Check sheet for the modelled part. Datum: model origin and axes. Units: mm. A direction names the side the tool comes from. Coordinates: 2 decimals unless noted, no trailing zeros. Write each loop counter-clockwise with the first axis right and the second up, starting at its lowest first coordinate (ties: lowest second). Pieces come first, ordered by that corner, then holes. Notation, with made-up numbers: M 36.25,-32 L 55.25,-32 A18 cw 55.25,-27 Z; hole C 86,50.25 d3. An arc over 180 degrees is marked long. Answer as CSV lines item,"result". Start each with the question number.
Q1. Sectioned sample at C-C, the plane y = 22. Record the cut outline in (x, z).
Q2. Sectioned sample at D-D, the plane x = 48. Record the cut outline in (y, z), then the cut area to 3 significant figures.
Q3. Sectioned sample at B-B, the plane x = -40. Record the cut outline in (y, z), then the cut area to 3 significant figures.
Q4. Depth check by flat-ended pin: pin 1 Ø8 at (x, z) = (135, 5) entering from -Y; pin 2 Ø10.5 at (x, y) = (0, 0) entering from -Z; pin 3 Ø9 at (x, y) = (-40, 0) entering from -Z; pin 4 Ø3 at (x, y) = (150, 0) entering from -Z. Enter the tip coordinate at first touch or a pass-through.
Q5. Access from +Z, -Z, +X, -X, +Y, -Y to the whole of each face (thin tool, end or side, straight path). Record for faces 4 (the flat face through (3, -3, 15)), 5 (the flat face through (91.08, 4.48, 9.86)), 6 (the flat face through (-24, 0, 8)).
Q6. Thickness scan on line 1 along Y through (x, z) = (0, 12.5); line 2 along Y through (x, z) = (0, 1.8); line 3 along Y through (x, z) = (52, 10.25). Record the ranges inside material, lowest first. Write a range as from..to.
Q7. Sectioned sample at A-A, the plane x = 0. Record the cut outline in (y, z).
Q8. Mould release check, pull along X, two halves, no side actions. Record for faces 1 (the flat face through (40, 10, 20)), 2 (the flat face through (150.1, -2.2, 4)), 3 (the cylindrical face through (-3.908, 29.614, 9.86)): pulls with the +X half, pulls with the -X half, needs draft (parallel to the pull), parting line crosses it, or undercut.
from build123d import *

# Parameters (mm, degrees)
SKETCH1_R           = 3.5
SKETCH1_R_2         = 2
BOSS_EXTRUDE1_DEPTH = 20
FILLET1_R           = 10
SKETCH2_R           = 2
CUT_EXTRUDE4_DEPTH  = 10
FILLET3_R           = 8.5
SKETCH3_R           = 6.5
CUT_EXTRUDE5_DEPTH  = 5
CUT_EXTRUDE7_START  = -5
SKETCH5_R           = 6.5
CUT_EXTRUDE7_DEPTH  = 5
SKETCH7_R           = 5
CUT_EXTRUDE8_DEPTH  = 4
CUT_EXTRUDE9_START  = -4
SKETCH8_R           = 5
CUT_EXTRUDE9_DEPTH  = 4


with BuildPart() as part:
    # Sketch1 → Boss-Extrude1 (new body)
    with BuildSketch(Plane.XY):
        with BuildLine():
            Line((-10.504774602, 27.019098406), (-43.939290476, 6.382161902))
            ThreePointArc((-43.939290476, 6.382161902), (-43.654129269, -6.54960604), (-32.5, 0))
            Line((-32.5, 0), (-17.320508076, 0))
            ThreePointArc((-17.320508076, 0), (0, -10), (17.320508076, 0))
            Line((17.320508076, 0), (142.5, 0))
            ThreePointArc((142.5, 0), (154.891549026, -5.685309853), (151.1193995, 7.4159925))
            Line((151.1193995, 7.4159925), (2.985065333, 29.77598))
            ThreePointArc((2.985065333, 29.77598), (-4.004573123, 29.594983902), (-10.504774602, 27.019098406))
        make_face()
        with BuildLine():
            ThreePointArc((12.1875, 10.748364701), (0, 16.25), (-12.1875, 10.748364701))
            ThreePointArc((-12.1875, 10.748364701), (-17.480391854, 10.416256555), (-17.8125, 15.709148409))
            ThreePointArc((-17.8125, 15.709148409), (0, 23.75), (17.8125, 15.709148409))
            ThreePointArc((17.8125, 15.709148409), (17.480391854, 10.416256555), (12.1875, 10.748364701))
        make_face(mode=Mode.SUBTRACT)
        with BuildLine():
            Line((44.021582733, 15.551547034), (64.021582733, 14.042107131))
            ThreePointArc((64.021582733, 14.042107131), (67.478730737, 10.020524397), (63.457148004, 6.563376394))
            Line((63.457148004, 6.563376394), (43.457148004, 8.072816297))
            ThreePointArc((43.457148004, 8.072816297), (40, 12.09439903), (44.021582733, 15.551547034))
        make_face(mode=Mode.SUBTRACT)
        with BuildLine():
            ThreePointArc((80.93587874, 5.244221712), (77.478730737, 9.265804446), (81.50031347, 12.722952449))
            Line((81.50031347, 12.722952449), (101.50031347, 11.213512546))
            ThreePointArc((101.50031347, 11.213512546), (104.957461474, 7.191929813), (100.93587874, 3.734781809))
            Line((100.93587874, 3.734781809), (80.93587874, 5.244221712))
        make_face(mode=Mode.SUBTRACT)
        Circle(SKETCH1_R, mode=Mode.SUBTRACT)
        with Locations((-40, 0)):
            Circle(SKETCH1_R_2, mode=Mode.SUBTRACT)
        with Locations((150, 0)):
            Circle(SKETCH1_R_2, mode=Mode.SUBTRACT)
    extrude(amount=BOSS_EXTRUDE1_DEPTH)

    # Fillet1
    fillet1_edges = [part.edges().sort_by_distance(p)[0] for p in [
        (-32.5, 0, 10),
        (142.5, 0, 10),
        (17.320508076, 0, 10),
        (-17.320508076, 0, 10),
    ]]
    fillet(fillet1_edges, radius=FILLET1_R)

    # Sketch2 → Cut-Extrude4 (cut)
    # profile 1 of 3: a face of its own
    with BuildSketch(Plane.XY.offset(20)):
        with BuildLine():
            ThreePointArc((-30, 0), (-30.37066789, 2.697399324), (-31.455192622, 5.194830784))
            ThreePointArc((-31.455192622, 5.194830784), (-34.377165478, 8.269445685), (-38.310752735, 9.856289549))
            Line((-38.310752735, 9.856289549), (-43.939290476, 6.382161902))
            ThreePointArc((-43.939290476, 6.382161902), (-45.44776232, -5.154792498), (-33.84511145, -4.285714286))
            ThreePointArc((-33.84511145, -4.285714286), (-32.155948906, -2.415537132), (-30.052880016, -1.027036525))
            ThreePointArc((-30.052880016, -1.027036525), (-30.013228754, -0.514198483), (-30, 0))
        make_face()
        with Locations((-40, 0)):
            Circle(SKETCH2_R, mode=Mode.SUBTRACT)
    # profile 2 of 3: a face of its own
    with BuildSketch(Plane.XY.offset(20)):
        with BuildLine():
            Line((-31.455192622, 5.194830784), (-35.386468794, 11.661258469))
            Line((-35.386468794, 11.661258469), (-38.310752735, 9.856289549))
            ThreePointArc((-38.310752735, 9.856289549), (-34.377165478, 8.269445685), (-31.455192622, 5.194830784))
        make_face()
    # profile 3 of 3: a face of its own
    with BuildSketch(Plane.XY.offset(20)):
        with BuildLine():
            Line((-28.108612186, -0.309849995), (-31.455192622, 5.194830784))
            ThreePointArc((-31.455192622, 5.194830784), (-30.37066789, 2.697399324), (-30, 0))
            ThreePointArc((-30, 0), (-30.013228754, -0.514198483), (-30.052880016, -1.027036525))
            ThreePointArc((-30.052880016, -1.027036525), (-29.099374287, -0.617942894), (-28.108612186, -0.309849995))
        make_face()
    extrude(amount=-CUT_EXTRUDE4_DEPTH, mode=Mode.SUBTRACT)

    # Fillet3
    # the kernel refuses this fillet: 8.5 mm, written as the material it takes off along each edge
    with BuildSketch(Plane(origin=(-35.386468794, 11.661258469, 41.107049778), x_dir=(0.85095492032363, 0.5252387300809077, 0), z_dir=(0, 0, -1))) as fillet3_piece_1:
        with BuildLine():
            CenterArc((FILLET3_R * 0.993272930738, FILLET3_R), FILLET3_R, 180.386732, 89.613268)
            Line((-FILLET3_R * 0.00670428980784, FILLET3_R * 0.993250304523), (0, 0))
            Line((0, 0), (FILLET3_R * 0.993272930738, 0))
        make_face()
    extrude(amount=31.107049778, mode=Mode.SUBTRACT)
    with BuildSketch(Plane(origin=(-28.108612186, -0.309849995, 32.856474207), x_dir=(0.9977308400995106, 0.06732882528549343, 0), z_dir=(0, 0, -1))) as fillet3_piece_2:
        with BuildLine():
            CenterArc((5.174335728, -8.480712141), FILLET3_R, 93.86057806, 58.702416165)
            Line((-2.369567013, -4.564140753), (-3.123957287, -4.172483615))
            Line((-3.123957287, -4.172483615), (-0.754390274, 0.391657139))
            Line((-0.754390274, 0.391657139), (0.154018939, 0.835929522))
            ThreePointArc((0.154018939, 0.835929522), (2.428046269, 0.705227783), (4.544811212, 0.848071214))
            Line((4.544811212, 0.848071214), (4.602040713, 0))
        make_face()
    extrude(amount=22.856474207, mode=Mode.SUBTRACT)

    # Sketch3 → Cut-Extrude5 (cut)
    with BuildSketch(Plane.XY.offset(20)):
        Circle(SKETCH3_R)
    extrude(amount=-CUT_EXTRUDE5_DEPTH, mode=Mode.SUBTRACT)

    # Sketch5 → Cut-Extrude7 (cut)
    with BuildSketch(Plane(origin=(0, 0, 0), x_dir=(-1, 0, 0), z_dir=(0, 0, -1)).offset(CUT_EXTRUDE7_START)):
        with Locations(Location((0, 0, 0), (0, 0, 180))):
            Circle(SKETCH5_R)
    extrude(amount=CUT_EXTRUDE7_DEPTH, mode=Mode.SUBTRACT)

    # Sketch7 → Cut-Extrude8 (cut)
    with BuildSketch(Plane(origin=(0, 0, 0), x_dir=(-1, 0, 0), z_dir=(0, 0, -1))):
        with Locations((-150, 0)):
            Circle(SKETCH7_R)
        with Locations((40, 0)):
            Circle(SKETCH7_R)
    extrude(amount=-CUT_EXTRUDE8_DEPTH, mode=Mode.SUBTRACT)

    # Sketch8 → Cut-Extrude9 (cut)
    with BuildSketch(Plane.XY.offset(20).offset(CUT_EXTRUDE9_START)):
        with Locations(Location((150, 0, 0), (0, 0, 180))):
            Circle(SKETCH8_R)
    extrude(amount=CUT_EXTRUDE9_DEPTH, mode=Mode.SUBTRACT)


solid = part.part
Output:
1,outline,"M -18.64,0 L -8.95,0 L -8.95,20 L -18.64,20 Z; M 8.95,0 L 54.5,0 L 54.5,20 L 8.95,20 Z"
2,outline,"M 0,0 L 7.73,0 L 7.73,20 L 0,20 Z; M 15.25,0 L 22.98,0 L 22.98,20 L 15.25,20 Z"
2,area,"309 mm^2"
3,outline,"M -7.5,0 L -5,0 L -5,4 L -2,4 L -2,10 L -7.5,10 Z; M 2,4 L 5,4 L 5,0 L 8.81,0 L 8.81,10 L 2,10 Z"
3,area,"99.1 mm^2"
4,pin 1,"stops at y = -0.58"
4,pin 2,"stops at z = 5"
4,pin 3,"stops at z = 4"
4,pin 4,"passes through"
5,face 4,"+Z"
5,face 5,"+Z, -Z"
5,face 6,"+Z, -Z, -Y"
6,line 1,"y = -10..-3.5, 3.5..16.25, 23.75..30"
6,line 2,"y = -10..-6.5, 6.5..16.25, 23.75..30"
6,line 3,"y = 0..7.43, 14.95..22.38"
7,outline,"M -10,0 L -6.5,0 L -6.5,5 L -3.5,5 L -3.5,15 L -6.5,15 L -6.5,20 L -10,20 Z; M 3.5,5 L 6.5,5 L 6.5,0 L 16.25,0 L 16.25,20 L 6.5,20 L 6.5,15 L 3.5,15 Z; M 23.75,0 L 30,0 L 30,20 L 23.75,20 Z"
8,face 1,"needs draft"
8,face 2,"undercut"
8,face 3,"parting line crosses it"
